Can you work these out from the model? Positions are in its coordinate system, mm. Face numbers are marked on the shaded views. A direction names the side the tool comes from. Coordinates: 2 decimals unless noted, no trailing zeros. Order: outer loops, then holes, each group sorted by start corner. A loop starts at its lowest first (then second) coordinate and runs counter-clockwise, first axis right, second up. Notation, with made-up numbers: (6, -6) -> (51, -6) arc R30 ccw to (51, 21) -> close; hole circle Ø7 at (43, 33.25). An arc over 180 degrees is marked (long way). Use a Markdown table: item, result. Add a question column.
1. For pin 1 Ø8 at (x, y) = (-11.5, 3) entering from -Z; pin 2 Ø2 at (y, z) = (1.5, 13) entering from -X; pin 3 Ø3.5 at (x, z) = (10.39, 6) entering from +Y, each with a flat end and sliding along its axis, tell me the tip position at first contact or that it passes through.
2. We'd pull the mould along X, two halves only. Please class the marked faces 4, 5, 6 and 7: pulls with the +X half, pulls with the -X half, needs draft (parallel to the pull), parting line crosses it, or undercut.
3. Suppose I cut it at A-A, the plane z = -12. List the corners of the cut face in (x, y) for me.
4. Suppose I cut it at B-B, the plane y = 1. List the corners of the cut face in (x, z) for me, then the cut area to 3 significant figures.
5. Suppose I cut it at C-C, the plane x = 0. List the corners of the cut face in (y, z) for me.
6. For the marked faces 1, 2 and 3, which set-ups out of +Z, -Z, +X, -X, +Y, -Y let a thin tool reach every point of the face, with its end or its side?
7. If I drill on line 1 along Z through (x, y) = (0, 1.7); line 2 along X through (y, z) = (0.65, 6); line 3 along Z through (x, y) = (1.25, 2.5), over which ranges is the centre line in solid material (lowest first)? Write a range as from..to.
8. Suppose I cut it at D-D, the plane z = -3.75. List the corners of the cut face in (x, y) for me, then the cut area to 3 significant figures.
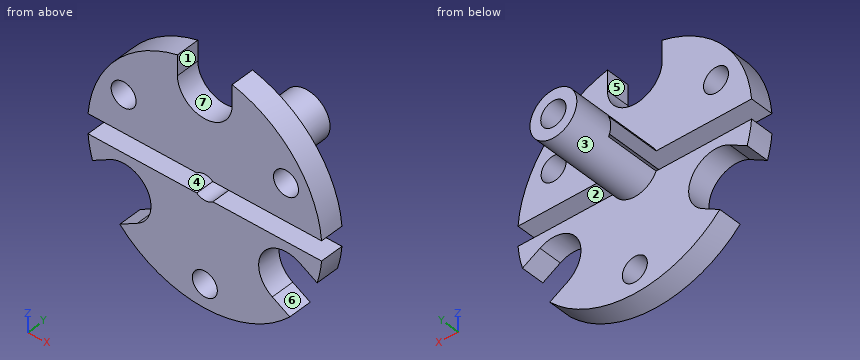
Autodesk Inventor part; units mm, degrees
ref_plane "YZ Plane" through (0, 0, 0) normal (1, 0, 0) x (0, 1, 0)
ref_plane "XZ Plane" through (0, 0, 0) normal (0, 1, 0) x (-1, 0, 0)
ref_plane "XY Plane" through (0, 0, 0) normal (0, 0, 1) x (1, 0, 0)
sketch "Sketch1" plane through (0, 0, 0) normal (0, 1, 0) x (-1, 0, 0)
  circle A0 centre (0, 0) radius 15
  dimension "d0" = 30
extrude "Extrusion1" add sketch "Sketch1" along normal blind 3
sketch "Sketch2" plane through (0, 3, 0) normal (0, 1, 0) x (1, 0, 0)
  circle A0 centre (0, 0) radius 12 construction
  point P0 (0, 12)
  point P1 (-10.3923, -6)
  point P2 (10.3923, -6)
  dimension "d3" = 24
  dimension "d4" = 120
hole "Hole1" at (0, 3, -12) at (-10.3923, 3, 6) at (10.3923, 3, 6) direction (0, -1, 0) diameter 3.2 end through all
sketch "Sketch4" plane through (0, 3, 0) normal (0, 1, 0) x (1, 0, 0)
  circle A0 centre (0, -12) radius 3.5
  circle A1 centre (0, 0) radius 15
  arc A2 (-3.5, -14.586) -> (3.5, -14.586) centre (0, 0) ccw
  line L0 (3.5, -12) -> (3.5, -14.586)
  line L1 (-3.5, -12) -> (-3.5, -14.586)
  dimension "d12" = 7
  dimension "d13" = 12
extrude "Extrusion2" cut sketch "Sketch4" against normal through all contours A0 A1 | L0 A1 A0 | A0 A1 L1 picked at (0.1406, -12.8318)
pattern_circular "Circular Pattern1" count 3 over 360 about axis through (0, 0, 0) along (0, 1, 0) of "Extrusion2"
sketch "Sketch6" plane through (0, 3, 0) normal (0, 1, 0) x (1, 0, 0)
  circle A0 centre (0, 0) radius 3
  dimension "d24" = 6
extrude "Extrusion4" add sketch "Sketch6" along normal blind 12
sketch "Sketch7" plane through (0, 0, 0) normal (0, -1, 0) x (1, 0, 0)
  line L0 (-1.5, 0) -> (63.9289, 0) construction
  line L1 (0, -1.5) -> (62.4289, -1.5)
  line L2 (62.4289, 1.5) -> (0, 1.5)
  arc A0 (0, 1.5) -> (0, -1.5) centre (0, 0) ccw
  arc A1 (62.4289, -1.5) -> (62.4289, 1.5) centre (62.4289, 0) ccw
  point P0 (31.2144, 0)
  dimension "d27" = 3
extrude "Extrusion5" [suppressed]
sketch "Sketch8" plane through (0, 15, 0) normal (0, 1, 0) x (1, 0, 0)
  point P0 (0, 0)
  point P1 (0, 0)
hole "Hole2" at (0, 15, 0) direction (0, -1, 0) diameter 3.242 end through all
sketch "Sketch9" plane through (0, 0, 0) normal (0, -1, 0) x (1, 0, 0)
  arc A0 (12.1423, -2.9689) -> (8.6423, -9.0311) centre (10.3923, -6) ccw
  line L0 (0, 0) -> (10.3923, -6) construction
  line L1 (0, 0) -> (9.8835, -17.1187) construction
  line L2 (0, 0) -> (17.8778, 0) construction
  line L3 (19.4334, 1) -> (1.2758, 1)
  circle A1 centre (0, 0) radius 1.621
  line L4 (-0.2281, -1.6049) -> (7.499, -14.9886)
  arc A2 (-10.8818, -10.3241) -> (10.8818, -10.3241) centre (0, 0) ccw
  arc A3 (14.3818, -4.2619) -> (3.5, 14.586) centre (0, 0) ccw
  arc A4 (6.6173, -13.4615) -> (14.9666, 1) centre (0, 0) ccw
  point P0 (10.8818, -10.3241)
  point P1 (14.3818, -4.2619)
  dimension "d37" = 30
  dimension "d38" = 30
  dimension "d39" = 1
  dimension "d40" = 1
extrude "Extrusion6" [suppressed]
fillet "Fillet1" [suppressed]
sketch "Sketch10" plane through (0, 0, 0) normal (0, -1, 0) x (1, 0, 0)
  arc A0 (14.3818, -4.2619) -> (3.5, 14.586) centre (0, 0) ccw
  line L0 (14.9478, -1.25) -> (-14.9478, -1.25)
  arc A1 (-3.5, 14.586) -> (-14.3818, -4.2619) centre (0, 0) ccw
  line L1 (-14.9478, 1.25) -> (14.9478, 1.25)
  arc A2 (-3.5, 14.586) -> (-14.3818, -4.2619) centre (0, 0) ccw
  arc A3 (14.9478, -1.25) -> (14.9478, 1.25) centre (0, 0) ccw
  arc A4 (-14.9478, 1.25) -> (-14.9478, -1.25) centre (0, 0) ccw
  dimension "d44" = 1.25
  dimension "d45" = 1.25
extrude "Extrusion7" cut sketch "Sketch10" against normal blind 10
equation "\"d38\" = d37"
equation "\"d40\" = d39"
properties part number "torsosc-support-flange-bottom-v2" material "Copper"
Worked out:
| question | item | result |
|---|---|---|
| 1 | pin 1 | stops at z = -12.99 |
| 1 | pin 2 | stops at x = -9 |
| 1 | pin 3 | stops at y = 3 |
| 2 | face 4 | needs draft |
| 2 | face 5 | undercut |
| 2 | face 6 | pulls with the +X half |
| 2 | face 7 | undercut |
| 3 | outline | (-9, 0) -> (-1.6, 0) -> (-1.6, 3) -> (-9, 3) -> close; (1.6, 0) -> (9, 0) -> (9, 3) -> (1.6, 3) -> close |
| 4 | outline | (-14.95, -1.25) arc R15 ccw to (-14.38, -4.26) -> (-12.14, -2.97) arc R3.5 cw to (-8.64, -9.03) -> (-10.88, -10.32) arc R15 ccw to (10.88, -10.32) -> (8.64, -9.03) arc R3.5 cw to (12.14, -2.97) -> (14.38, -4.26) arc R15 ccw to (14.95, -1.25) -> (1.03, -1.25) arc R1.62 cw to (-1.03, -1.25) -> close; (-14.95, 1.25) -> (-1.03, 1.25) arc R1.62 cw to (1.03, 1.25) -> (14.95, 1.25) arc R15 ccw to (3.5, 14.59) -> (3.5, 12) arc R3.5 cw to (-3.5, 12) -> (-3.5, 14.59) arc R15 ccw to start; hole circle Ø3.2 at (-10.39, 6); hole circle Ø3.2 at (0, -12); hole circle Ø3.2 at (10.39, 6) |
| 4 | area | 489 mm² |
| 5 | outline | (0, -15) -> (3, -15) -> (3, -13.6) -> (0, -13.6) -> close; (0, -10.4) -> (3, -10.4) -> (3, -3) -> (15, -3) -> (15, -1.62) -> (0, -1.62) -> close; (0, 1.62) -> (15, 1.62) -> (15, 3) -> (3, 3) -> (3, 8.5) -> (0, 8.5) -> close |
| 6 | face 1 | +Z, +Y, -Y |
| 6 | face 2 | +X, -X, -Y |
| 6 | face 3 | +Y |
| 7 | line 1 | z = -15..-13.6, -10.4..-1.62, 1.62..8.5 |
| 7 | line 2 | x = -13.75..-11.99, -8.79..8.79, 11.99..13.75 |
| 7 | line 3 | z = -14.95..-13, -11..-1.25, 1.25..8.73 |
| 8 | outline | (-14.52, 0) -> (-13.5, 0) -> (-13.5, 3) -> (-14.52, 3) -> close; (-7.71, 0) -> (7.71, 0) -> (7.71, 3) -> (-7.71, 3) -> close; (13.5, 0) -> (14.52, 0) -> (14.52, 3) -> (13.5, 3) -> close |
| 8 | area | 52.4 mm² |
